from build123d import *

# Parameters (mm, degrees)
F0_R     = 7.9375
F0_R_2   = 6.985
F1_DEPTH = 2.54
F2_R     = 0.508


# Not quite as in the source:
# - a fillet or chamfer that OpenCascade refuses, or shapes differently, is made with other operations: its cross-section is extruded or revolved along the edge and cut away or added


with BuildPart() as f1:
    # F0 (on Front) → F1 (new body)
    with BuildSketch(Plane.XZ):
        Circle(F0_R)
        Circle(F0_R_2, mode=Mode.SUBTRACT)
    extrude(amount=F1_DEPTH)

    # F2
    f2_edges = [f1.edges().sort_by_distance(p)[0] for p in [
        (-7.9375, -2.54, 0),
        (-7.9375, 0, 0),
    ]]
    fillet(f2_edges, radius=F2_R)

    # F3: fillet of radius 0.508 on 2 edges, made by hand

    # F3_s1 → F3_t2 (revolve, cut)
    with BuildSketch(Plane.XY):
        with BuildLine():
            ThreePointArc((7.4295, 0), (7.112, -0.1680052083), (6.985, -0.5040156248))
            Line((6.985, -0.5040156248), (6.985, 0))
            Line((6.985, 0), (7.4295, 0))
        make_face()
    revolve(axis=Axis((0, 0, 0), (0, -1, 0)), mode=Mode.SUBTRACT)

    # F3_s3 → F3_t4 (revolve, cut)
    with BuildSketch(Plane.XY):
        with BuildLine():
            ThreePointArc((7.4295, -2.54), (7.112, -2.3719947917), (6.985, -2.0359843752))
            Line((6.985, -2.0359843752), (6.985, -2.54))
            Line((6.985, -2.54), (7.4295, -2.54))
        make_face()
    revolve(axis=Axis((0, -2.54, 0), (0, -1, 0)), mode=Mode.SUBTRACT)


solid = f1.part
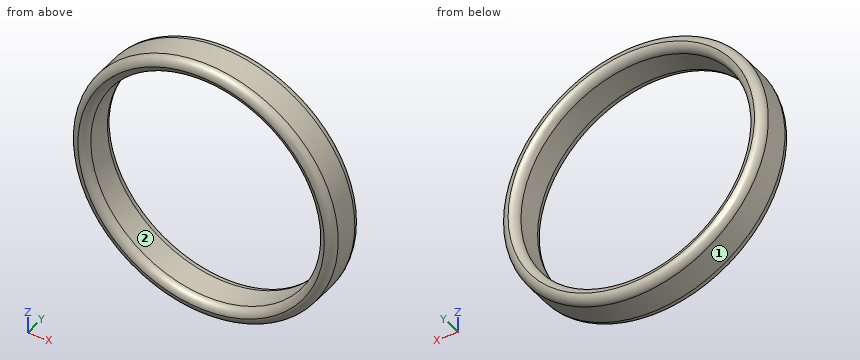
Model file for the job. Use its own axes, mm. Face numbers are marked on the shaded views. Round coordinates to 2 decimals unless told otherwise and drop trailing zeros. Order: outer loops, then holes, each group sorted by start corner. A loop starts at its lowest first (then second) coordinate and runs counter-clockwise, first axis right, second up. Notation, with made-up numbers: M 47.25,-37 L 86.25,-37 A19 ccw 86.25,-3 Z; hole C -33,89 d2. An arc over 180 degrees is marked long. Write each question's results on one line, items separated by ' | '. Start each with the question number.
(1) Saw through at B-B, the plane x = 0. Give the cut face in (y, z) (1 decimal), then the cut area to 3 significant figures.
(2) Drop flat-ended pins along their axis: pin 1 (1 mm diameter, centred on y = -1, z = 3.5, fed in from -X); pin 2 (1 mm diameter, centred on y = -1.5, z = -5, fed in from +X); pin 3 (1 mm diameter, centred on y = -1, z = -4.5, fed in from +X). Give the stop position or say it passes through.
(3) Saw through at A-A, the plane z = 0. Give the cut face in (x, y) (1 decimal).
(4) Probe probe 1 along Z at (x, y) = (0, -1.2) (1 decimal); probe 2 along X at (y, z) = (-0.35, 1.25); probe 3 along Z at (x, y) = (3, -1.5). List the from-to ranges inside material, lowest first. Write a range as from..to.
(5) Two-plate mould, pull along X, no slides. Class the marked faces 1 and 2: pulls with the +X half, pulls with the -X half, needs draft (parallel to the pull), parting line crosses it, or undercut.
(6) Saw through at C-C, the plane y = -0.85. Give the cut face in (x, z) (1 decimal).
Established:
1) outline: M -2.5,-7.4 A0.5 ccw -2,-7.9 L -0.5,-7.9 A0.5 ccw 0,-7.4 A0.5 ccw -0.5,-7 L -2,-7 A0.5 ccw Z; M -2.5,7.4 A0.5 ccw -2,7 L -0.5,7 A0.5 ccw 0,7.4 A0.5 ccw -0.5,7.9 L -2,7.9 A0.5 ccw Z | area: 4.40 mm^2
2) pin 1: stops at x = -7.35 | pin 2: stops at x = 6.54 | pin 3: stops at x = 6.86
3) outline: M -7.9,-2 A0.5 ccw -7.4,-2.5 A0.5 ccw -7,-2 L -7,-0.5 A0.5 ccw -7.4,0 A0.5 ccw -7.9,-0.5 Z; M 7,-2 A0.5 ccw 7.4,-2.5 A0.5 ccw 7.9,-2 L 7.9,-0.5 A0.5 ccw 7.4,0 A0.5 ccw 7,-0.5 Z
4) probe 1: z = -7.9..-7, 7..7.9 | probe 2: x = -7.81..-6.9, 6.9..7.81 | probe 3: z = -7.35..-6.31, 6.31..7.35
5) face 1: parting line crosses it | face 2: undercut
6) outline: C 0,0 d15.9; hole C 0,0 d14
